Source: CAD feature listing. Evaluate the final solid. Frame: model axes, mm. A direction names the side the tool comes from. Coordinates: 2 decimals unless noted, no trailing zeros. Order: outer loops, then holes, each group sorted by start corner. A loop starts at its lowest first (then second) coordinate and runs counter-clockwise, first axis right, second up.
```python
from build123d import *

# Parameters (mm, degrees)
SKETCH1_W           = 70
SKETCH1_H           = 121.1
SKETCH1_R           = 3.25
SKETCH1_W_2         = 54
SKETCH1_H_2         = 105.1
BOSS_EXTRUDE1_DEPTH = 5
SKETCH2_W           = 5
SKETCH2_H           = 121.1
BOSS_EXTRUDE2_DEPTH = 2
SKETCH3_W           = 5
SKETCH3_H           = 72
BOSS_EXTRUDE3_DEPTH = 2
SKETCH4_W           = 5
SKETCH4_H           = 123.1
BOSS_EXTRUDE4_DEPTH = 2
SKETCH5_W           = 5
SKETCH5_H           = 74
BOSS_EXTRUDE5_DEPTH = 2


with BuildPart() as part:
    # Sketch1 → Boss-Extrude1 (new body)
    with BuildSketch(Plane(origin=(0, 0, 0), x_dir=(0, 0, -1), z_dir=(1, 0, 0))):
        Rectangle(SKETCH1_W, SKETCH1_H)
        with Locations((-31, -56.55)):
            Circle(SKETCH1_R, mode=Mode.SUBTRACT)
        with Locations(Location((31, -56.55, 0), (0, 0, 180))):
            Circle(SKETCH1_R, mode=Mode.SUBTRACT)
        with Locations((-31, 55.45)):
            Circle(SKETCH1_R, mode=Mode.SUBTRACT)
        with Locations(Location((31, 55.45, 0), (0, 0, 180))):
            Circle(SKETCH1_R, mode=Mode.SUBTRACT)
        Rectangle(SKETCH1_W_2, SKETCH1_H_2, mode=Mode.SUBTRACT)
    extrude(amount=BOSS_EXTRUDE1_DEPTH)

    # Sketch2 → Boss-Extrude2 (add)
    with BuildSketch(Plane.XY.offset(35)):
        with Locations((2.5, 0)):
            Rectangle(SKETCH2_W, SKETCH2_H)
    extrude(amount=BOSS_EXTRUDE2_DEPTH)

    # Sketch3 → Boss-Extrude3 (add)
    with BuildSketch(Plane(origin=(0, 60.55, 0), x_dir=(1, 0, 0), z_dir=(0, 1, 0))):
        with Locations((2.5, -1)):
            Rectangle(SKETCH3_W, SKETCH3_H)
    extrude(amount=BOSS_EXTRUDE3_DEPTH)

    # Sketch4 → Boss-Extrude4 (add)
    with BuildSketch(Plane(origin=(0, 0, -35), x_dir=(-1, 0, 0), z_dir=(0, 0, -1))):
        with Locations((-2.5, 1)):
            Rectangle(SKETCH4_W, SKETCH4_H)
    extrude(amount=BOSS_EXTRUDE4_DEPTH)

    # Sketch5 → Boss-Extrude5 (add)
    with BuildSketch(Plane.XZ.offset(60.55)):
        with Locations((2.5, 0)):
            Rectangle(SKETCH5_W, SKETCH5_H)
    extrude(amount=BOSS_EXTRUDE5_DEPTH)


solid = part.part
```
Q1. Set-up query: faces 1 (the flat face through (2, 1, -37)), 2 (the flat face through (2, -52.55, 0)). Return all of +Z, -Z, +X, -X, +Y, -Y with unobstructed straight access to the full face (end or side cutting, diameter ignored); none if empty.
Solutions:
face 1: -Z, +X, -X, +Y, -Y
face 2: +X, -X
Q2. Pull-direction query (Y, two-part tool) for faces 3 (the flat face through (2, -62.55, 1)), 4 (the flat face through (3, 62.55, 1)), 5 (the flat face through (0, 0.3, 27.2)), 6 (the cylindrical face through (2.465, -53.667, -29.5)); classes: pulls with the +Y half, pulls with the -Y half, needs draft (parallel to the pull), parting line crosses it, or undercut.
Solutions:
face 3: pulls with the -Y half
face 4: pulls with the +Y half
face 5: needs draft
face 6: undercut
Q3. Section query C-C on y = 10. Output: boundary loops of the cut face in (x, z), plus the area to 3 significant figures.
Solutions:
outline: (0, -37) - (5, -37) - (5, -27) - (0, -27) - close; (0, 27) - (5, 27) - (5, 37) - (0, 37) - close
area: 100 mm2
Q4. Section query D-D on z = -31. Output: boundary loops of the cut face in (x, y).
Solutions:
outline: (0, -62.55) - (5, -62.55) - (5, -59.8) - (0, -59.8) - close; (0, -53.3) - (5, -53.3) - (5, 52.2) - (0, 52.2) - close; (0, 58.7) - (5, 58.7) - (5, 62.55) - (0, 62.55) - close
Q5. Section query B-B on y = -56.55. Output: boundary loops of the cut face in (x, z).
Solutions:
outline: (0, -37) - (5, -37) - (5, -34.25) - (0, -34.25) - close; (0, -27.75) - (5, -27.75) - (5, 27.75) - (0, 27.75) - close; (0, 34.25) - (5, 34.25) - (5, 37) - (0, 37) - close
Q6. Material intervals for line 1 along Y through (x, z) = (1.8, -31); line 2 along Z through (x, y) = (1.1, 16.5); line 3 along Y through (x, z) = (4.05, 15), sorted ascending.
Solutions:
line 1: y = -62.55 to -59.8, -53.3 to 52.2, 58.7 to 62.55
line 2: z = -37 to -27, 27 to 37
line 3: y = -62.55 to -52.55, 52.55 to 62.55
Q7. Section query A-A on z = -6.5. Output: boundary loops of the cut face in (x, y), plus the area to 3 significant figures.
Solutions:
outline: (0, -62.55) - (5, -62.55) - (5, -52.55) - (0, -52.55) - close; (0, 52.55) - (5, 52.55) - (5, 62.55) - (0, 62.55) - close
area: 100 mm2
Q8. Pin query (flat end, axial travel): P1, Ø8.5, axis at y = -56.55, z = 31, coming from the -X side. Return the tip coordinate at first contact, or that it passes through.
Solutions:
P1: stops at x = 0
